Can you work these out from the model? Positions are in its coordinate system, mm. Give positions to 0.01 mm unless a question says otherwise; leave off trailing zeros. Write each loop counter-clockwise with the first axis right and the second up, starting at its lowest first coordinate (ties: lowest second). Pieces come first, ordered by that corner, then holes. Notation, with made-up numbers: (57.25, 20.5) -> (64.25, 20.5) arc R31 ccw to (64.25, 52.5) -> close; hole circle Ø11 at (8.5, 86). An arc over 180 degrees is marked (long way). One line per item, written item: value.
Autodesk Inventor part; units mm, degrees
ref_plane "YZ Plane" through (0, 0, 0) normal (1, 0, 0) x (0, 1, 0)
ref_plane "XZ Plane" through (0, 0, 0) normal (0, 1, 0) x (-1, 0, 0)
ref_plane "XY Plane" through (0, 0, 0) normal (0, 0, 1) x (1, 0, 0)
sketch "Skizze1" plane through (0, 0, 0) normal (0, 0, 1) x (1, 0, 0)
  line L0 (0, 0) -> (127, 0)
  line L1 (127, 0) -> (127, 37.5)
  line L2 (127, 37.5) -> (0, 37.5)
  line L3 (0, 37.5) -> (0, 0)
  line L4 (4.75, 3.65) -> (14.75, 3.65)
  line L5 (14.75, 3.65) -> (14.75, 13.85)
  line L6 (14.75, 13.85) -> (4.75, 13.85)
  line L7 (4.75, 13.85) -> (4.75, 3.65)
  line L8 (4.75, 33.85) -> (4.75, 23.65)
  line L9 (14.75, 33.85) -> (4.75, 33.85)
  line L10 (14.75, 23.65) -> (14.75, 33.85)
  line L11 (4.75, 23.65) -> (14.75, 23.65)
  line L12 (26.25, 13.85) -> (26.25, 3.65)
  line L13 (36.25, 13.85) -> (26.25, 13.85)
  line L14 (36.25, 3.65) -> (36.25, 13.85)
  line L15 (26.25, 3.65) -> (36.25, 3.65)
  line L16 (26.25, 33.85) -> (26.25, 23.65)
  line L17 (36.25, 33.85) -> (26.25, 33.85)
  line L18 (36.25, 23.65) -> (36.25, 33.85)
  line L19 (26.25, 23.65) -> (36.25, 23.65)
  line L20 (47.75, 13.85) -> (47.75, 3.65)
  line L21 (57.75, 13.85) -> (47.75, 13.85)
  line L22 (57.75, 3.65) -> (57.75, 13.85)
  line L23 (47.75, 3.65) -> (57.75, 3.65)
  line L24 (47.75, 33.85) -> (47.75, 23.65)
  line L25 (57.75, 33.85) -> (47.75, 33.85)
  line L26 (57.75, 23.65) -> (57.75, 33.85)
  line L27 (47.75, 23.65) -> (57.75, 23.65)
  line L28 (69.25, 13.85) -> (69.25, 3.65)
  line L29 (79.25, 13.85) -> (69.25, 13.85)
  line L30 (79.25, 3.65) -> (79.25, 13.85)
  line L31 (69.25, 3.65) -> (79.25, 3.65)
  line L32 (69.25, 33.85) -> (69.25, 23.65)
  line L33 (79.25, 33.85) -> (69.25, 33.85)
  line L34 (79.25, 23.65) -> (79.25, 33.85)
  line L35 (69.25, 23.65) -> (79.25, 23.65)
  line L36 (90.75, 13.85) -> (90.75, 3.65)
  line L37 (100.75, 13.85) -> (90.75, 13.85)
  line L38 (100.75, 3.65) -> (100.75, 13.85)
  line L39 (90.75, 3.65) -> (100.75, 3.65)
  line L40 (90.75, 33.85) -> (90.75, 23.65)
  line L41 (100.75, 33.85) -> (90.75, 33.85)
  line L42 (100.75, 23.65) -> (100.75, 33.85)
  line L43 (90.75, 23.65) -> (100.75, 23.65)
  line L44 (112.25, 13.85) -> (112.25, 3.65)
  line L45 (122.25, 13.85) -> (112.25, 13.85)
  line L46 (122.25, 3.65) -> (122.25, 13.85)
  line L47 (112.25, 3.65) -> (122.25, 3.65)
  line L48 (112.25, 33.85) -> (112.25, 23.65)
  line L49 (122.25, 33.85) -> (112.25, 33.85)
  line L50 (122.25, 23.65) -> (122.25, 33.85)
  line L51 (112.25, 23.65) -> (122.25, 23.65)
  line L52 (0, 18.75) -> (40, 18.75)
  line L53 (40, 18.75) -> (40, 28.75)
  line L54 (40, 28.75) -> (60, 28.75)
  line L55 (60, 28.75) -> (60, 23.75)
  arc A0 (60, 23.75) -> (65, 18.75) centre (65, 23.75) ccw
  line L56 (65, 18.75) -> (127, 18.75)
  arc A1 (23.2272, 0) -> (17.7728, 0) centre (20.5, -1.25) ccw
  line L57 (0, 17.5) -> (40, 17.5)
  line L58 (40, 17.5) -> (40, 18.75)
  line L59 (127, 17.5) -> (65, 17.5)
  arc A2 (60, 22.5) -> (65, 17.5) centre (65, 22.5) ccw
  line L60 (60, 22.5) -> (60, 23.75)
  point P0 (63.5, 37.5)
  point P1 (42, 18.75)
  point P2 (85, 18.75)
  point P3 (63.5, 0)
  point P4 (55, 23.75)
  point P5 (52.46, 23.75)
  point P6 (49.92, 23.75)
  point P7 (47.38, 23.75)
  point P8 (55, 21.21)
  point P9 (52.46, 21.21)
  point P10 (49.92, 21.21)
  point P11 (47.38, 21.21)
  point P12 (55, 18.67)
  point P13 (52.46, 18.67)
  point P14 (49.92, 18.67)
  point P15 (47.38, 18.67)
  point P16 (31.25, 3.65)
  point P17 (4.75, 8.75)
  dimension "d0" = 127
  dimension "d1" = 37.5
  dimension "d2" = 10.2
  dimension "d3" = 10
  dimension "d6" = 20
  dimension "d9" = 21.5
  dimension "d13" = 5.75
  dimension "d17" = 43
  dimension "d18" = 21.5
  dimension "d19" = 28.75
  dimension "d20" = 60
  dimension "d21" = 5
  dimension "d22" = 20
  dimension "d24" = 5
  dimension "d36" = 2.54
  dimension "d39" = 2.54
  dimension "d43" = 3
  dimension "d44" = 1.25
  dimension "d45" = 10.75
  dimension "d48" = 8.75
  dimension "d49" = 8.75
  dimension "d50" = 5
extrude "Extrusion1" add sketch "Skizze1" along normal blind 1 contours L3 L57 L58 L53 L54 L24 L27 L26 L55 L60 A2 L59 L1 L0 A1 | L54 L26 L27 L24
fillet "Rundung1" radius 5 2 edges at (127, 0, 0.5) (0, 0, 0.5)
hole "Bohrung1" at (55, 23.75, 0) at (55, 21.21, 0) at (52.46, 21.21, 0) at (49.92, 21.21, 0) at (49.92, 23.75, 0) at (52.46, 23.75, 0) at (55, 18.67, 0) at (52.46, 18.67, 0) at (49.92, 18.67, 0) at (47.38, 18.67, 0) at (47.38, 21.21, 0) at (47.38, 23.75, 0) direction (0, 0, 1) diameter 1.4 end through all
fillet "Rundung2" radius 2 2 edges at (60, 28.75, 0.5) (40, 28.75, 0.5)
fillet "Rundung3" radius 5 2 edges at (127, 17.5, 0.5) (0, 17.5, 0.5)
fillet "Rundung4" radius 3 2 edges at (17.7728, 0, 0.5) (23.2272, 0, 0.5)
sketch "Skizze2" plane through (0, 0, 1) normal (0, 0, 1) x (1, 0, 0)
  arc A0 (0, 5) -> (5, 0) centre (5, 5) ccw
  line L0 (5, 0) -> (16.2647, 0)
  arc A1 (122, 0) -> (127, 5) centre (122, 5) ccw
  line L1 (127, 5) -> (127, 12.5)
  line L2 (0, 12.5) -> (0, 5)
  line L3 (112.25, 13.85) -> (122.25, 13.85)
  line L4 (122.25, 13.85) -> (122.25, 3.65)
  line L5 (122.25, 3.65) -> (112.25, 3.65)
  line L6 (112.25, 3.65) -> (112.25, 13.85)
  line L7 (90.75, 13.85) -> (100.75, 13.85)
  line L8 (100.75, 13.85) -> (100.75, 3.65)
  line L9 (100.75, 3.65) -> (90.75, 3.65)
  line L10 (90.75, 3.65) -> (90.75, 13.85)
  line L11 (69.25, 13.85) -> (79.25, 13.85)
  line L12 (79.25, 13.85) -> (79.25, 3.65)
  line L13 (79.25, 3.65) -> (69.25, 3.65)
  line L14 (69.25, 3.65) -> (69.25, 13.85)
  line L15 (47.75, 13.85) -> (57.75, 13.85)
  line L16 (57.75, 13.85) -> (57.75, 3.65)
  line L17 (57.75, 3.65) -> (47.75, 3.65)
  line L18 (47.75, 3.65) -> (47.75, 13.85)
  line L19 (26.25, 13.85) -> (36.25, 13.85)
  line L20 (36.25, 13.85) -> (36.25, 3.65)
  line L21 (36.25, 3.65) -> (26.25, 3.65)
  line L22 (26.25, 3.65) -> (26.25, 13.85)
  line L23 (4.75, 3.65) -> (4.75, 13.85)
  line L24 (4.75, 13.85) -> (14.75, 13.85)
  line L25 (14.75, 13.85) -> (14.75, 3.65)
  line L26 (14.75, 3.65) -> (4.75, 3.65)
  line L27 (60, 22.5) -> (60, 26.75)
  line L28 (58, 28.75) -> (42, 28.75)
  line L29 (40, 26.75) -> (40, 17.5)
  arc A2 (60, 26.75) -> (58, 28.75) centre (58, 26.75) ccw
  arc A3 (42, 28.75) -> (40, 26.75) centre (42, 26.75) ccw
  circle A4 centre (55, 23.75) radius 0.7
  arc A5 (22.6176, 0.875) -> (18.3824, 0.875) centre (20.5, -1.25) ccw
  line L30 (24.7353, 0) -> (122, 0)
  arc A6 (22.6176, 0.875) -> (24.7353, 0) centre (24.7353, 3) ccw
  arc A7 (16.2647, 0) -> (18.3824, 0.875) centre (16.2647, 3) ccw
  line L31 (122, 17.5) -> (65, 17.5)
  arc A8 (60, 22.5) -> (65, 17.5) centre (65, 22.5) ccw
  line L32 (40, 17.5) -> (5, 17.5)
  arc A9 (127, 12.5) -> (122, 17.5) centre (122, 12.5) ccw
  arc A10 (5, 17.5) -> (0, 12.5) centre (5, 12.5) ccw
  circle A11 centre (47.38, 18.67) radius 0.7
  circle A12 centre (47.38, 21.21) radius 0.7
  circle A13 centre (47.38, 23.75) radius 0.7
  circle A14 centre (49.92, 23.75) radius 0.7
  circle A15 centre (49.92, 21.21) radius 0.7
  circle A16 centre (49.92, 18.67) radius 0.7
  circle A17 centre (52.46, 18.67) radius 0.7
  circle A18 centre (52.46, 21.21) radius 0.7
  circle A19 centre (52.46, 23.75) radius 0.7
  circle A20 centre (55, 21.21) radius 0.7
  circle A21 centre (55, 18.67) radius 0.7
  point P0 (0, 0)
properties part number "bat_contacts_v2_plate_contact" material "Kupfer"
1) If we section it at B-B (x = 96.5): Write out the boundary of the cut face in (y, z).
Answer list:
outline: (0, 0) -> (3.65, 0) -> (3.65, 1) -> (0, 1) -> close; (13.85, 0) -> (17.5, 0) -> (17.5, 1) -> (13.85, 1) -> close
2) I need wall thicknesses on L1, parallel to Y at x = 52.46, z = 0.5; L2, parallel to Y at x = 47.38, z = 0.3; L3, parallel to Y at x = 70.5, z = 0.55. Which ranges of each line are inside material? Lowest first, please.
Answer list:
L1: y = 0 to 3.65, 13.85 to 17.97, 19.37 to 20.51, 21.91 to 23.05, 24.45 to 28.75
L2: y = 0 to 17.97, 19.37 to 20.51, 21.91 to 23.05, 24.45 to 28.75
L3: y = 0 to 3.65, 13.85 to 17.5
3) If we section it at A-A (y = 11): Write out the boundary of the cut face in (x, z).
Answer list:
outline: (0, 0) -> (4.75, 0) -> (4.75, 1) -> (0, 1) -> close; (14.75, 0) -> (26.25, 0) -> (26.25, 1) -> (14.75, 1) -> close; (36.25, 0) -> (47.75, 0) -> (47.75, 1) -> (36.25, 1) -> close; (57.75, 0) -> (69.25, 0) -> (69.25, 1) -> (57.75, 1) -> close; (79.25, 0) -> (90.75, 0) -> (90.75, 1) -> (79.25, 1) -> close; (100.75, 0) -> (112.25, 0) -> (112.25, 1) -> (100.75, 1) -> close; (122.25, 0) -> (127, 0) -> (127, 1) -> (122.25, 1) -> close
4) Will this pin go through, and if not, where does the flat tip stop? pin 1 (0.5 mm diameter, centred on x = 25.5, z = 0.5, fed in from +Y).
Answer list:
pin 1: stops at y = 17.5
5) If we section it at C-C (z = 0.65): State how many separate pieces and enclosed holes the cut face has, and give its area (3 significant figures).
Answer list:
separate pieces: 1
enclosed holes: 18
area: 1,790 mm^2
